from build123d import *

# Parameters (mm, degrees)
ESQUISSE1_R             = 2.5
BOSS_EXTRU_1_DEPTH      = 16
ESQUISSE2_R             = 4.25
BOSS_EXTRU_2_DEPTH      = 5
ENL_V_MAT_EXTRU_1_DEPTH = 3.5


with BuildPart() as part:
    # Esquisse1 → Boss.-Extru.1 (new body)
    with BuildSketch(Plane(origin=(0, 0, 0), x_dir=(0, 0, -1), z_dir=(1, 0, 0))):
        Circle(ESQUISSE1_R)
    extrude(amount=BOSS_EXTRU_1_DEPTH)

    # Esquisse2 → Boss.-Extru.2 (add)
    with BuildSketch(Plane(origin=(16, 0, 0), x_dir=(0, 0, -1), z_dir=(1, 0, 0))):
        Circle(ESQUISSE2_R)
    extrude(amount=BOSS_EXTRU_2_DEPTH)

    # Esquisse3 → Enlèv. mat.-Extru.1 (cut)
    with BuildSketch(Plane(origin=(21, 0, 0), x_dir=(0, 0, -1), z_dir=(1, 0, 0))):
        Polygon((2.309401077, 0), (1.154700538, 2), (-1.154700538, 2), (-2.309401077, 0), (-1.154700538, -2), (1.154700538, -2), align=None)
    extrude(amount=-ENL_V_MAT_EXTRU_1_DEPTH, mode=Mode.SUBTRACT)


solid = part.part
Can you work these out from the model? Positions are in its coordinate system, mm. A direction names the side the tool comes from. Coordinates: 2 decimals unless noted, no trailing zeros. Loops run counter-clockwise (first coordinate to the right, second up) from the corner with the lowest first, then second, coordinate; pieces in that order, holes last. Notation, with made-up numbers: M 85.5,46 L 108.5,46 A25 cw 108.5,72 Z; hole C -23,89.25 d3. An arc over 180 degrees is marked long. Return JSON: item names as keys, results as strings. Group by question number.
Item 1: Imagine slicing it at D-D (y = -3.25). Please give me the cut outline in (x, z), and give its area (3 significant figures).
Item 2: Imagine slicing it at C-C (x = 3.25). Please give me the cut outline in (y, z), and give its area (3 significant figures).
Item 3: I'm going to push flat-ended pins straight in: pin 1 Ø1 at (x, y) = (10, 1.5) entering from +Z; pin 2 Ø1.5 at (x, z) = (6, 0.5) entering from -Y; pin 3 Ø4 at (x, z) = (7.5, -2) entering from +Y. Where does each tip first touch, or does it pass through?
Item 4: Imagine slicing it at A-A (z = 0). Please give me the cut outline in (x, y).
Item 5: Thinking about a two-plate mould opening in Z: for faces 4 (the cylindrical face through (18.465, 3.584, -2.285)), 5 (the flat face through (16, -2, -2)), 6 (the flat face through (19.27, -0.99, 1.74)), which applies, released by +Z, released by -Z, zero draft, split by the parting line, or undercut?
Item 6: Imagine slicing it at B-B (y = -1). Please give me the cut outline in (x, z), and give its area (3 significant figures).
Item 7: If I drill on L1, parallel to Z at x = 14.5, y = -1.5; L2, parallel to Y at x = 19.25, z = -0.5; L3, parallel to X at y = 1.5, z = 0.25, over which ranges is the centre line in solid material (lowest first)? Write a range as from..to.
Item 8: On a 3-axis mill with a long thin cutter (end or side, diameter ignored), from which of +Z, -Z, +X, -X, +Y, -Y can I reach the whole of each face in a straight line? I mean faces 1 (the flat face through (19.27, 0.99, -1.74)), 2 (the flat face through (21, -1, -2)), 3 (the cylindrical face through (7.89, -2.44, 0.54)). Say none if no direction works.
Verdict:
{
 "1": {"outline": "M 16,-2.74 L 21,-2.74 L 21,2.74 L 16,2.74 Z", "area": "27.4 mm^2"},
 "2": {"outline": "C 0,0 d5", "area": "19.6 mm^2"},
 "3": {"pin 1": "stops at z = 2.29", "pin 2": "stops at y = -2.5", "pin 3": "stops at y = 2.5"},
 "4": {"outline": "M 0,-2.5 L 16,-2.5 L 16,-4.25 L 21,-4.25 L 21,-2 L 17.5,-2 L 17.5,2 L 21,2 L 21,4.25 L 16,4.25 L 16,2.5 L 0,2.5 Z"},
 "5": {"face 4": "split by the parting line", "face 5": "zero draft", "face 6": "undercut"},
 "6": {"outline": "M 0,-2.29 L 16,-2.29 L 16,-4.13 L 21,-4.13 L 21,-1.73 L 17.5,-1.73 L 17.5,1.73 L 21,1.73 L 21,4.13 L 16,4.13 L 16,2.29 L 0,2.29 Z", "area": "103 mm^2"},
 "7": {"L1": "z = -2..2", "L2": "y = -4.22..-2, 2..4.22", "L3": "x = 0..17.5"},
 "8": {"face 1": "+X", "face 2": "+Z, -Z, +X, +Y, -Y", "face 3": "-X"}
}
